from build123d import *

# Parameters (mm, degrees)
F0_R     = 10.9728
F1_DEPTH = 2.0066
F2_R     = 5.207
F3_DEPTH = 1.524
F4_R     = 4.0005
F5_DEPTH = 4.1148
F8_DEPTH = 2.54


with BuildPart() as f1:
    # F0 (on Top) → F1 (new body)
    with BuildSketch(Plane.XY):
        Circle(F0_R)
    extrude(amount=F1_DEPTH)

    # F2 (on face) → F3 (join)
    with BuildSketch(Plane(origin=(0, 0, 0), x_dir=(1, 0, 0), z_dir=(0, 0, -1))):
        Circle(F2_R)
    extrude(amount=F3_DEPTH)

    # F4 (on Top) → F5 (join)
    with BuildSketch(Plane.XY):
        Circle(F4_R)
    extrude(amount=-F5_DEPTH)

    # F7 (on face) → F8 (join)
    with BuildSketch(Plane.XY):
        Polygon((4.283191, 6.165847), (0, 18.501436), (-3.597881, 6.165847), (-18.332055, 6.165847), (-6.681778, 0), (-10.79364, -15.078778), (0, -6.169742), (10.79364, -15.078778), (7.709743, 0), (17.304089, 6.165847), align=None)
    extrude(amount=F8_DEPTH)


solid = f1.part
Could you check a few things on this model? Use its own coordinates, in mm. A direction names the side the tool comes from. Give positions to 0.01 mm unless a question says otherwise; leave off trailing zeros. Loops run counter-clockwise (first coordinate to the right, second up) from the corner with the lowest first, then second, coordinate; pieces in that order, holes last. Notation, with made-up numbers: (72.5, 27) -> (83.5, 27) arc R31 ccw to (83.5, 66) -> close; hole circle Ø9 at (28, 18.5). An arc over 180 degrees is marked (long way). Answer as CSV lines item,"result". Start each with the question number.
(1) Which directions (+Z, -Z, +X, -X, +Y, -Y) give clear straight access to the entire face, cutting with the end or side of a thin tool? Please do faces 4 (the flat face through (-5, 8, 2.007)), 5 (the flat face through (-1, 6, 0)), 6 (the flat face through (9.616, -9.32, 1.534)).
(2) If we section it at B-B on y = -9.5: Write out the boundary of the cut face in (x, z).
(3) If we section it at A-A on x = 9.5: Write out the boundary of the cut face in (y, z), then the cut area to 3 significant figures.
(4) If we section it at C-C on z = 1.5: Write out the boundary of the cut face in (x, y) (3 decimals), then the cut area to 3 significant figures.
(5) We'd pull the mould along Y, two halves only. Please class faces 1 (the cylindrical face through (10.71, -2.39, 0.99)), 2 (the flat face through (-6.7, -11.7, 1.5)), 3 (the flat face through (2, 4, -1.524)): released by +Y, released by -Y, zero draft, split by the parting line, or undercut.
(6) If we section it at D-D on y = 1: Write out the boundary of the cut face in (x, z), then the cut area to 3 significant figures.
(7) I'm going to push flat-ended pins straight in: pin 1 Ø1.5 at (x, z) = (-12.5, 1.5) entering from +Y; pin 2 Ø3 at (x, y) = (11, 6.5) entering from -Z; pin 3 Ø3 at (x, z) = (-9.5, 1) entering from +Y. Where does each tip first touch, or does it pass through?
(8) I need wall thicknesses on probe 1 along Z at (x, y) = (-10.5, 2.5); probe 2 along X at (y, z) = (-9, 2.25); probe 3 along X at (y, z) = (-2, 1.5). Which ranges of each line are inside material? Lowest first, please.
Computed:
1,face 4,"+Z, -X, +Y"
1,face 5,"-Z"
1,face 6,"+Z, +X"
2,outline,"(-9.27, 0) -> (9.65, 0) -> (9.65, 2.54) -> (4.03, 2.54) -> (4.03, 2.01) -> (-4.03, 2.01) -> (-4.03, 2.54) -> (-9.27, 2.54) -> close"
3,outline,"(-14.01, 0) -> (-8.75, 0) -> (-8.75, 2.54) -> (-14.01, 2.54) -> close; (-5.49, 0) -> (6.17, 0) -> (6.17, 2.54) -> (1.15, 2.54) -> (1.15, 2.01) -> (-5.49, 2.01) -> close"
3,area,"39.4 mm2"
4,outline,"(-18.332, 6.166) -> (-10.759, 2.158) arc R10.973 ccw to (-8.555, -6.871) -> (-10.794, -15.079) -> (-4.596, -9.964) arc R10.973 ccw to (4.596, -9.964) -> (10.794, -15.079) -> (8.995, -6.284) arc R10.973 ccw to (10.792, 1.981) -> (17.304, 6.166) -> (9.077, 6.166) arc R10.973 ccw to (2.734, 10.627) -> (0, 18.501) -> (-2.265, 10.737) arc R10.973 ccw to (-9.077, 6.166) -> close"
4,area,"471 mm2"
5,face 1,"undercut"
5,face 2,"released by -Y"
5,face 3,"zero draft"
6,outline,"(-10.93, 0) -> (-5.11, 0) -> (-5.11, -1.52) -> (-3.87, -1.52) -> (-3.87, -4.11) -> (3.87, -4.11) -> (3.87, -1.52) -> (5.11, -1.52) -> (5.11, 0) -> (10.93, 0) -> (10.93, 2.01) -> (9.27, 2.01) -> (9.27, 2.54) -> (-8.57, 2.54) -> (-8.57, 2.01) -> (-10.93, 2.01) -> close"
6,area,"89.0 mm2"
7,pin 1,"stops at y = 6.17"
7,pin 2,"stops at z = 0"
7,pin 3,"stops at y = 7.51"
8,probe 1,"z = 0 to 2.54"
8,probe 2,"x = -9.14 to -3.43, 3.43 to 9.55"
8,probe 3,"x = -10.79 to 10.79"
